Design review of the part shown in the three views and the two pictorial views. Dimensions are in mm from the part's minimum x, y and z. A direction names the side the tool comes from. Coordinates: 2 decimals unless noted, no trailing zeros. Write each loop counter-clockwise with the first axis right and the second up, starting at its lowest first coordinate (ties: lowest second). Pieces come first, ordered by that corner, then holes. Notation, with made-up numbers: (53, 66) -> (69, 66) arc R22 ccw to (69, 94) -> close; hole circle Ø11 at (18.25, 28.25). An arc over 180 degrees is marked (long way). Write each question's results on one line, items separated by ' | '.
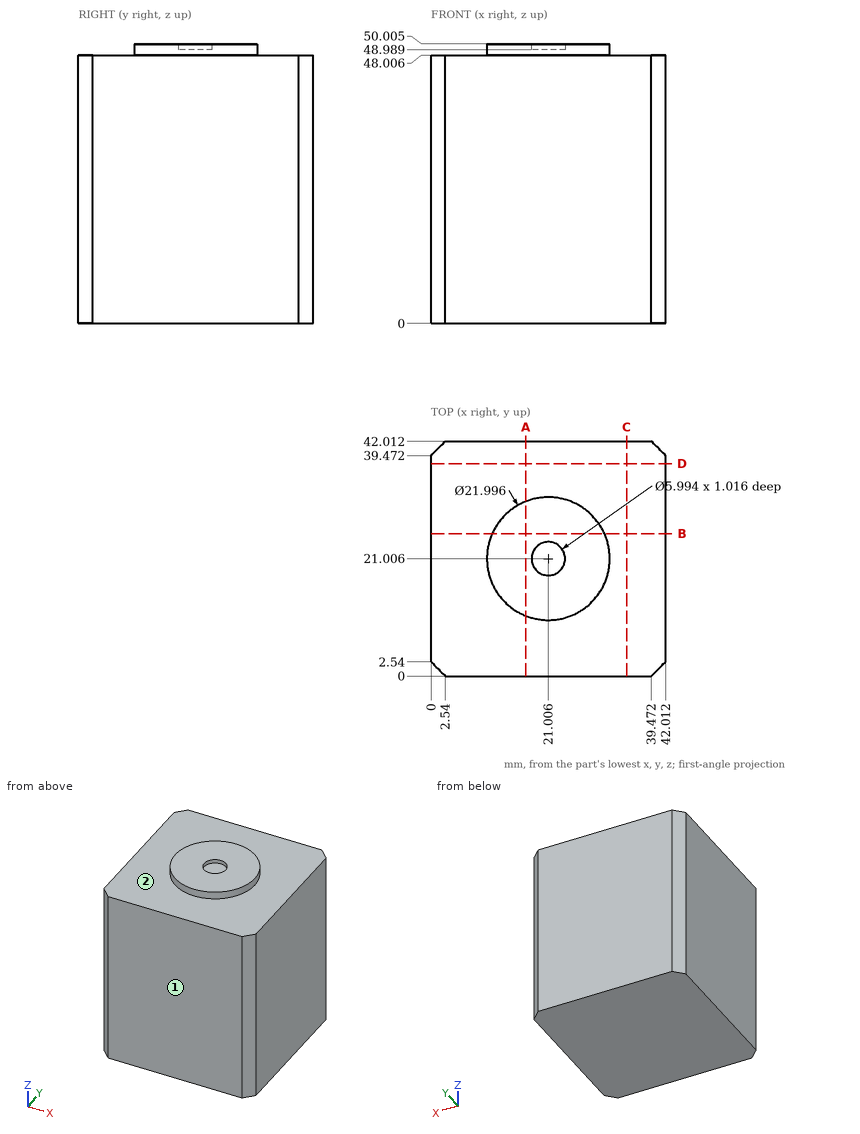
Q1. Machinability: for the marked faces 1 and 2, which of the approach directions +Z, -Z, +X, -X, +Y, -Y give a long, thin tool a straight path to every point of the face, cutting with its end or side? Answer none if there is none.
Solution:
face 1: +Z, -Z, +X, -X, -Y | face 2: +Z
Q2. Add section C-C (x = 35). Write out the cut boundary in (y, z), plus the area to 3 significant figures.
Solution:
outline: (0, 0) -> (42.01, 0) -> (42.01, 48.01) -> (0, 48.01) -> close | area: 2,020 mm²
Q3. Add section B-B (y = 25.5). Write out the cut boundary in (x, z) (1 decimal), plus the area to 3 significant figures.
Solution:
outline: (0, 0) -> (42, 0) -> (42, 48) -> (31, 48) -> (31, 50) -> (11, 50) -> (11, 48) -> (0, 48) -> close | area: 2,060 mm²
Q4. For line 1 (Z direction, x = 19, y = 33); line 2 (Z direction, x = 19, y = 21); line 3 (Y direction, x = 40, z = 29) (1 decimal), list the stretches that pass through material, from the lowest coordinate up. Write a range as from..to.
Solution:
line 1: 0..48.01 | line 2: 0..48.99 | line 3: 0.5..41.5
Q5. Add section A-A (x = 17). Write out the cut boundary in (y, z) (1 decimal), plus the area to 3 significant figures.
Solution:
outline: (0, 0) -> (42, 0) -> (42, 48) -> (31.2, 48) -> (31.2, 50) -> (10.8, 50) -> (10.8, 48) -> (0, 48) -> close | area: 2,060 mm²
